Read the model definition and answer for the solid it produces. Units are mm, in the model's axes. A direction names the side the tool comes from. Coordinates: 2 decimals unless noted, no trailing zeros. Loops run counter-clockwise (first coordinate to the right, second up) from the corner with the lowest first, then second, coordinate; pieces in that order, holes last. Notation, with made-up numbers: (-13, 30.5) - (-3, 30.5) arc R33 cw to (-3, 65.5) - close; hole circle Ø10 at (-27.5, 23.5). An arc over 180 degrees is marked (long way). Use one line per item in the form item = value.
from build123d import *

# Parameters (mm, degrees)
MM_1_D              = 6
MM_1_DEPTH          = 4
MM_1_TIP            = 1.802581857
CUT_EXTRUDE_1_DEPTH = 4
FILLET_1_R          = 0.2
CHAMFER_1_SIZE      = 0.6
FILLET_2_R          = 0.4


with BuildPart() as part:
    # 草图1 → 旋转1 (revolve)
    with BuildSketch(Plane.XY):
        Polygon((0, 0), (0, 6.5), (8, 6.5), (8, 4), (28, 4), (28, 0), align=None)
    revolve(axis=Axis((0, 0, 0), (1, 0, 0)))

    # 大小mm 暗销孔1
    with Locations(Plane.ZY):
        with Locations((0, 0)):
            Hole(MM_1_D / 2, depth=MM_1_DEPTH)
            with Locations((0, 0, -(MM_1_DEPTH + MM_1_TIP / 2))):  # 118° drill point
                Cone(0, MM_1_D / 2, MM_1_TIP, mode=Mode.SUBTRACT)

    # 草图4 → 切除-拉伸1 (cut)
    with BuildSketch(Plane.ZY):
        Polygon((3, 1.732050808), (0, 3.464101615), (-3, 1.732050808), (-3, -1.732050808), (0, -3.464101615), (3, -1.732050808), align=None)
    extrude(amount=-CUT_EXTRUDE_1_DEPTH, mode=Mode.SUBTRACT)

    # 圆角1
    fillet_1_edges = [part.edges().sort_by_distance(p)[0] for p in [
        (0, -6.5, 0),
    ]]
    fillet(fillet_1_edges, radius=FILLET_1_R)

    # 倒角1
    chamfer_1_edges = [part.edges().sort_by_distance(p)[0] for p in [
        (28, -4, 0),
    ]]
    chamfer(chamfer_1_edges, length=CHAMFER_1_SIZE)

    # 圆角2
    fillet_2_edges = [part.edges().sort_by_distance(p)[0] for p in [
        (8, -4, 0),
    ]]
    fillet(fillet_2_edges, radius=FILLET_2_R)


solid = part.part
Item 1: Find the intervals of material crossed by L1, parallel to X at y = 5.5, z = -3; L2, parallel to Z at x = 10.25, y = 0; L3, parallel to Z at x = 12.5, y = -2, in increasing order.
Results below:
L1 = 0 to 8
L2 = -4 to 4
L3 = -3.46 to 3.46
Item 2: The part is cut by section A-A on x = 3.5. Give the vertices of the cut face in (y, z), plus the area to 3 significant figures.
Results below:
outline = circle Ø13 at (0, 0); hole (-3.46, 0) - (-1.73, -3) - (1.73, -3) - (3.46, 0) - (1.73, 3) - (-1.73, 3) - close
area = 102 mm²
Item 3: Each of these flat-tipped pins is pushed along its axis until it touches: P1, Ø0.8, axis at y = -1.5, z = -2.5, coming from the -X side; P2, Ø4, axis at x = 13, y = -0.5, coming from the -Z side; P3, Ø1.5, axis at x = 21.5, z = 3, coming from the -Y side. Where does it stop, or does it pass through?
Results below:
P1 = 4
P2 = -4
P3 = -3.31
Item 4: Which of the six approach directions +Z, -Z, +X, -X, +Y, -Y give full straight-line access (tool end or side, diameter ignored) to faces 4 (the flat face through (2, 2.6, -1.5)), 5 (the flat face through (0, 2.9, -1.3)), 6 (the cylindrical face through (18.033, -0.867, -3.905))?
Results below:
face_4 = -X
face_5 = +Z, -Z, -X, +Y, -Y
face_6 = +X
Item 5: The part is cut by section B-B on x = 11.5. Give the vertices of the cut face in (y, z), plus the area to 3 significant figures.
Results below:
outline = circle Ø8 at (0, 0)
area = 50.3 mm²
Item 6: For a pull along Y with two mould halves and no side action, classify faces 1 (the flat face through (2, 0, -3)), 2 (the cylindrical face through (4.155, -5.158, -3.955)), 3 (the flat face through (28, 0, 0)) as +Y half, -Y half, draft (parallel to the pull), parting line (faces both ways), or undercut.
Results below:
face_1 = undercut
face_2 = parting line
face_3 = draft
